```python
from build123d import *

# Parameters (mm, degrees)
SKETCH_1_W          = 100
SKETCH_1_H          = 100
EXTRUDE_1_DEPTH     = 3
EXTRUDE_2_DEPTH     = 32
SKETCH_3_R          = 9
EXTRUDE_3_DEPTH     = 3
SKETCH_4_W          = 60
SKETCH_4_H          = 10
CUT_EXTRUDE_1_DEPTH = 2.5
CHAMFER_1_SIZE      = 2


with BuildPart() as part:
    # Эскиз1 → Бобышка-Вытянуть1 (new body)
    with BuildSketch(Plane(origin=(0, 0, 0), x_dir=(1, 0, 0), z_dir=(0, 1, 0))):
        with Locations((-19.913614773, -13.668080108)):
            Rectangle(SKETCH_1_W, SKETCH_1_H)
    extrude(amount=EXTRUDE_1_DEPTH)

    # Эскиз2 → Бобышка-Вытянуть2 (add)
    with BuildSketch(Plane(origin=(0, 3, 0), x_dir=(1, 0, 0), z_dir=(0, 1, 0))):
        Polygon((27.586385227, -61.041825342), (27.586385227, -63.668080108), (30.086385227, -63.668080108), (30.086385227, 36.331919892), (-69.913614773, 36.331919892), (-69.913614773, -63.668080108), (-67.413614773, -63.668080108), (-67.413614773, -61.041825342), (-67.413614773, 33.831919892), (27.586385227, 33.831919892), align=None)
    extrude(amount=EXTRUDE_2_DEPTH)

    # Эскиз3 → Бобышка-Вытянуть3 (add)
    with BuildSketch(Plane(origin=(0, 3, 0), x_dir=(1, 0, 0), z_dir=(0, 1, 0))):
        with Locations((-10.839314865, 25.657938065)):
            Circle(SKETCH_3_R)
        with Locations((-59.962592759, 25.657938065)):
            Circle(SKETCH_3_R)
        with Locations((-59.962592759, -32.348529185)):
            Circle(SKETCH_3_R)
        with Locations(Location((-10.839314865, -32.348529185, 0), (0, 0, 270))):
            Circle(SKETCH_3_R)
    extrude(amount=EXTRUDE_3_DEPTH)

    # Эскиз4 → Вырез-Вытянуть1 (cut)
    with BuildSketch(Plane.ZY.offset(69.913614773)):
        with Locations((5.326629647, 11.873940314)):
            Rectangle(SKETCH_4_W, SKETCH_4_H)
    extrude(amount=-CUT_EXTRUDE_1_DEPTH, mode=Mode.SUBTRACT)

    # Фаска1
    chamfer_1_edges = [part.edges().sort_by_distance(p)[0] for p in [
        (-67.413614773, 3, 50.53230301),
        (27.586385227, 3, 14.918080108),
        (10.256751916, 3, -33.831919892),
        (-35.400953812, 3, -33.831919892),
        (-67.413614773, 3, 3.34529556),
    ]]
    chamfer(chamfer_1_edges, length=CHAMFER_1_SIZE)


solid = part.part
```
CAD build for the part. Positions are in the model's coordinates, mm. A direction names the side the tool comes from. Give positions to 0.01 mm unless a question says otherwise; leave off trailing zeros. Write each loop counter-clockwise with the first axis right and the second up, starting at its lowest first coordinate (ties: lowest second). Pieces come first, ordered by that corner, then holes. Notation, with made-up numbers: M 66,28 L 120,28 A29 cw 120,56 Z; hole C 88,-8 d6. An arc over 180 degrees is marked long. Return JSON: item names as keys, results as strings. Group by question number.
(1) 3-axis set-ups, long thin cutter, end or side, ignore diameter. For faces 4 (the face through (-59, 6, 32)), 5 (the face through (-21, 0, 13)), 6 (the face through (-14.29, 4.48, 40.66)), 7 (the face through (-69, 12, -24.673)), 8 (the face through (-69.914, 17.3, 14.4)): which of +Z, -Z, +X, -X, +Y, -Y reach the whole face in a straight line?
(2) Band-saw the part on D-D (y = 28.5). Give the cut face in (x, z), and give its area (4 significant figures).
(3) Band-saw the part on C-C (x = -24). Give the cut face in (y, z), and give its area (3 significant figures).
(4) Band-saw the part on A-A (y = 10). Give the cut face in (x, z), and give its area (4 significant figures).
(5) Flat gauge pins, fed straight in: pin 1 Ø12 at (x, y) = (-33, 15) entering from +Z; pin 2 Ø0.9 at (x, z) = (-65, -32.5) entering from +Y. Where does each tip first touch, or does it go through?
(6) Drill centre lines: L1, parallel to X at y = 24.5, z = 20; L2, parallel to Y at x = -20.5, z = 9; L3, parallel to Z at x = -46.5, y = 8. Where is each one in solid material? Low to high. Write a range as [from, to].
(7) Band-saw the part on B-B (z = 19). Give the cut face in (x, y), and give its area (3 significant figures).
(8) Mould opens along Z. For faces 1 (the face through (-69, 16.874, 5)), 2 (the face through (-19, 17, -36.332)), 3 (the face through (-11, 6, -25)) say: pulls with the +Z half, pulls with the -Z half, needs draft (parallel to the pull), parting line crosses it, or undercut.
Entries:
{
 "1": {"face 4": "+Z, +Y", "face 5": "+Z, -Z, +X, -X, -Y", "face 6": "+Y", "face 7": "-X", "face 8": "+Z, -Z, -X, +Y, -Y"},
 "2": {"outline": "M -69.91,-36.33 L 30.09,-36.33 L 30.09,63.67 L 27.59,63.67 L 27.59,-33.83 L -67.41,-33.83 L -67.41,63.67 L -69.91,63.67 Z", "area": "737.5 mm^2"},
 "3": {"outline": "M 0,-36.33 L 35,-36.33 L 35,-33.83 L 5,-33.83 L 3,-31.83 L 3,63.67 L 0,63.67 Z", "area": "382 mm^2"},
 "4": {"outline": "M -69.91,-36.33 L 30.09,-36.33 L 30.09,63.67 L 27.59,63.67 L 27.59,-33.83 L -67.41,-33.83 L -67.41,-24.67 L -69.91,-24.67 Z; M -69.91,35.33 L -67.41,35.33 L -67.41,63.67 L -69.91,63.67 Z", "area": "587.5 mm^2"},
 "5": {"pin 1": "stops at z = -33.83", "pin 2": "stops at y = 6"},
 "6": {"L1": "x = [-69.91, -67.41], [27.59, 30.09]", "L2": "y = [0, 3]", "L3": "z = [-36.33, -33.83]"},
 "7": {"outline": "M -69.91,0 L 30.09,0 L 30.09,35 L 27.59,35 L 27.59,5 L 25.59,3 L -65.41,3 L -67.41,5 L -67.41,6.87 L -69.91,6.87 Z; M -69.91,16.87 L -67.41,16.87 L -67.41,35 L -69.91,35 Z", "area": "439 mm^2"},
 "8": {"face 1": "undercut", "face 2": "pulls with the -Z half", "face 3": "needs draft"}
}
